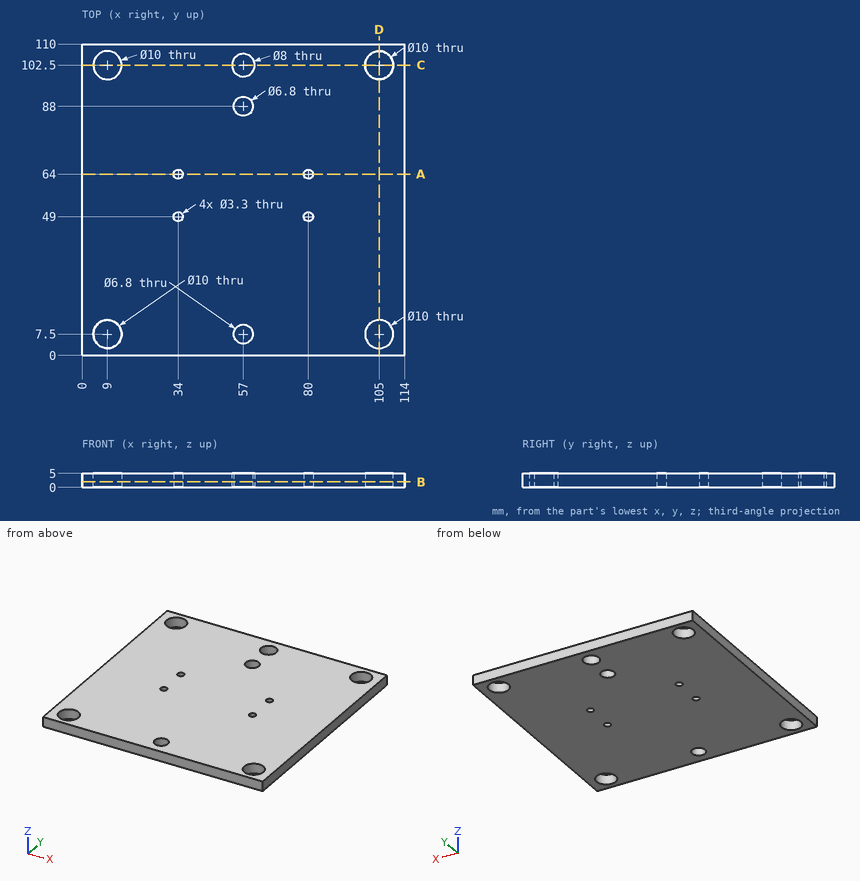
The figure shows three views and two pictorial views of one solid part (mm, origin at its lowest corner). Answer the questions. Give positions to 0.01 mm unless a question says otherwise; leave off trailing zeros. Order: outer loops, then holes, each group sorted by start corner. A loop starts at its lowest first (then second) coordinate and runs counter-clockwise, first axis right, second up. Notation, with made-up numbers: M 19,82 L 57,82 A37 ccw 57,120 Z; hole C 49,70 d3. An arc over 180 degrees is marked long. Return JSON: item names as keys, results as strings.
1) Straight lines are drawn through the part: line 1 along Y through (x, z) = (34, 1.3); line 2 along Y through (x, z) = (105, 1.25); line 3 along X through (y, z) = (64, 3.15). For each, find the intervals that lie inside material, in ascending order. Write a range as [from, to].
Resolved:
{"line 1": "[0, 47.35], [50.65, 62.35], [65.65, 110]", "line 2": "[0, 2.5], [12.5, 97.5], [107.5, 110]", "line 3": "[0, 32.35], [35.65, 78.35], [81.65, 114]"}
2) Section D-D, the plane x = 105 is taken. Write down the section's boundary in (y, z), plus the area to 3 significant figures.
Resolved:
{"outline": "M 0,0 L 2.5,0 L 2.5,5 L 0,5 Z; M 12.5,0 L 97.5,0 L 97.5,5 L 12.5,5 Z; M 107.5,0 L 110,0 L 110,5 L 107.5,5 Z", "area": "450 mm^2"}
3) Section C-C, the plane y = 102.5 is taken. Write down the section's boundary in (x, z), plus the area to 3 significant figures.
Resolved:
{"outline": "M 0,0 L 4,0 L 4,5 L 0,5 Z; M 14,0 L 53,0 L 53,5 L 14,5 Z; M 61,0 L 100,0 L 100,5 L 61,5 Z; M 110,0 L 114,0 L 114,5 L 110,5 Z", "area": "430 mm^2"}
4) Section B-B, the plane z = 1.95 is taken. Give the number of separate pieces and of enclosed holes in the cut face, plus the area to 3 significant figures.
Resolved:
{"separate pieces": "1", "enclosed holes": "11", "area": "12,100 mm^2"}
5) Section A-A, the plane y = 64 is taken. Write down the section's boundary in (x, z).
Resolved:
{"outline": "M 0,0 L 32.35,0 L 32.35,5 L 0,5 Z; M 35.65,0 L 78.35,0 L 78.35,5 L 35.65,5 Z; M 81.65,0 L 114,0 L 114,5 L 81.65,5 Z"}
